Geometry: final body of the model. Coordinates: model frame, mm. A direction names the side the tool comes from. Round coordinates to 2 decimals unless told otherwise and drop trailing zeros. Order: outer loops, then holes, each group sorted by start corner. A loop starts at its lowest first (then second) coordinate and runs counter-clockwise, first axis right, second up. Notation, with made-up numbers: (65.25, 62) -> (104.25, 62) arc R9 ccw to (104.25, 71) -> close; hole circle Ø6 at (48.25, 71). An arc over 180 degrees is marked (long way). Put each result on its own line as item: value.
```python
from build123d import *

# Parameters (mm, degrees)
EXTRUDE_1_DEPTH = 10
CHAMFER_1_SIZE  = 1


with BuildPart() as part:
    # 草图1 → 拉伸-薄壁1 (new body)
    with BuildSketch(Plane.XY):
        with BuildLine():
            Line((14.631143099, -58.188741623), (2.394484263, -4.446228189))
            ThreePointArc((2.394484263, -4.446228189), (0.089779865, 5.049201875), (-2.551037445, -4.358291862))
            Line((-2.551037445, -4.358291862), (-14.631143099, -58.188741623))
            Line((-14.631143099, -58.188741623), (-19.509807266, -57.09391929))
            Line((-19.509807266, -57.09391929), (-8.04810956, -6.019172079))
            ThreePointArc((-8.04810956, -6.019172079), (0.106256457, 10.049438271), (7.919038593, -6.187998688))
            Line((7.919038593, -6.187998688), (19.506366852, -57.078699572))
            Line((19.506366852, -57.078699572), (14.631143099, -58.188741623))
        make_face()
    extrude(amount=EXTRUDE_1_DEPTH)

    # 倒角1
    chamfer_1_edges = [part.edges().sort_by_distance(p)[0] for p in [
        (19.506366852, -57.078699572, 5),
        (14.631143099, -58.188741623, 5),
        (-14.631143099, -58.188741623, 5),
        (-8.591090272, -31.273516742, 10),
        (-19.509807266, -57.09391929, 5),
        (0.089779865, 5.049201875, 10),
        (8.512813681, -31.317484906, 10),
        (17.068754976, -57.633720597, 10),
        (13.712702723, -31.63334913, 10),
        (0.106256457, 10.049438271, 10),
        (-13.778958413, -31.556545684, 10),
        (0.106256457, 10.049438271, 0),
        (13.712702723, -31.63334913, 0),
        (17.068754976, -57.633720597, 0),
        (8.512813681, -31.317484906, 0),
        (0.089779865, 5.049201875, 0),
        (-17.070475183, -57.641330456, 10),
        (-8.591090272, -31.273516742, 0),
        (-17.070475183, -57.641330456, 0),
        (-13.778958413, -31.556545684, 0),
    ]]
    chamfer(chamfer_1_edges, length=CHAMFER_1_SIZE)


solid = part.part
```
1. Contact query for flat-ended pins moving along their axis: P1, Ø6, axis at y = -22, z = 4.5, coming from the +X side; P2, Ø3, axis at y = -13, z = 5.5, coming from the -X side; P3, Ø1.5, axis at x = -4, z = 1, coming from the +Y side. Output: stop coordinate, or through.
Ans:
P1: x = 12.2
P2: x = -9.95
P3: y = 9.51
2. Set-up query: faces 4 (the face through (8.486, -31.199, 4.944)), 5 (the face through (8.98, -31.087, 9.507)), 6 (the face through (12.97, -30.67, 0.49)). Return all of +Z, -Z, +X, -X, +Y, -Y with unobstructed straight access to the full face (end or side cutting, diameter ignored); none if empty.
Ans:
face 4: +Z, -Z, -Y
face 5: +Z, -Y
face 6: -Z, +X
3. Cut plane C-C on x = 13. Return loops of the section in (y, z).
Ans:
outline: (-51.02, 1) -> (-46.52, 0) -> (-33.01, 0) -> (-28.5, 1) -> (-28.5, 9) -> (-33.01, 10) -> (-46.52, 10) -> (-51.02, 9) -> close
4. Cut plane D-D on x = 0. Return loops of the section in (y, z), and give its area (3 significant figures).
Ans:
outline: (5.05, 1) -> (6.05, 0) -> (9.05, 0) -> (10.05, 1) -> (10.05, 9) -> (9.05, 10) -> (6.05, 10) -> (5.05, 9) -> close
area: 48.0 mm²
5. Cut plane B-B on z = 3. Return loops of the section in (x, y).
Ans:
outline: (-19.29, -56.12) -> (-18.53, -57.31) -> (-15.61, -57.97) -> (-14.41, -57.21) -> (-2.55, -4.36) arc R5.05 cw (long way) to (2.39, -4.45) -> (14.41, -57.21) -> (15.61, -57.97) -> (18.53, -57.3) -> (19.28, -56.1) -> (7.92, -6.19) arc R10.05 ccw (long way) to (-8.05, -6.02) -> close
6. Draft query along X for faces 1 (the face through (-0.19, 9.21, 9.84)), 2 (the face through (-15.02, -57.6, 4.94)), 3 (the face through (-16.94, -57.15, 9.51)). Return one class per face: +X half, -X half, draft (parallel to the pull), parting line (faces both ways), or undercut.
Ans:
face 1: parting line
face 2: undercut
face 3: -X half
7. Cut plane A-A on y = 0. Return loops of the section in (x, z).
Ans:
outline: (-10.05, 1) -> (-9.05, 0) -> (-6.05, 0) -> (-5.05, 1) -> (-5.05, 9) -> (-6.05, 10) -> (-9.05, 10) -> (-10.05, 9) -> close; (5.05, 1) -> (6.05, 0) -> (9.05, 0) -> (10.05, 1) -> (10.05, 9) -> (9.05, 10) -> (6.05, 10) -> (5.05, 9) -> close
8. Material intervals for probe 1 along X at (y, z) = (0, 6); probe 2 along Y at (x, z) = (0, 3.5); probe 3 along X at (y, z) = (-54, 2.5), sorted ascending.
Ans:
probe 1: -10.05 to -5.05, 5.05 to 10.05
probe 2: 5.05 to 10.05
probe 3: -18.82 to -13.69, 13.68 to 18.81
